Source: three-view drawing plus pictorial views. Frame: mm from the lowest corner of the part. Give positions to 0.01 mm unless a question says otherwise; leave off trailing zeros. Order: outer loops, then holes, each group sorted by start corner. A loop starts at its lowest first (then second) coordinate and runs counter-clockwise, first axis right, second up. Notation, with made-up numbers: M -0.5,69 L 20.5,69 A26 cw 20.5,90 Z; hole C 29.25,7 d3. An arc over 180 degrees is marked long. Use CSV: the item, a comma, the result in double quotes.
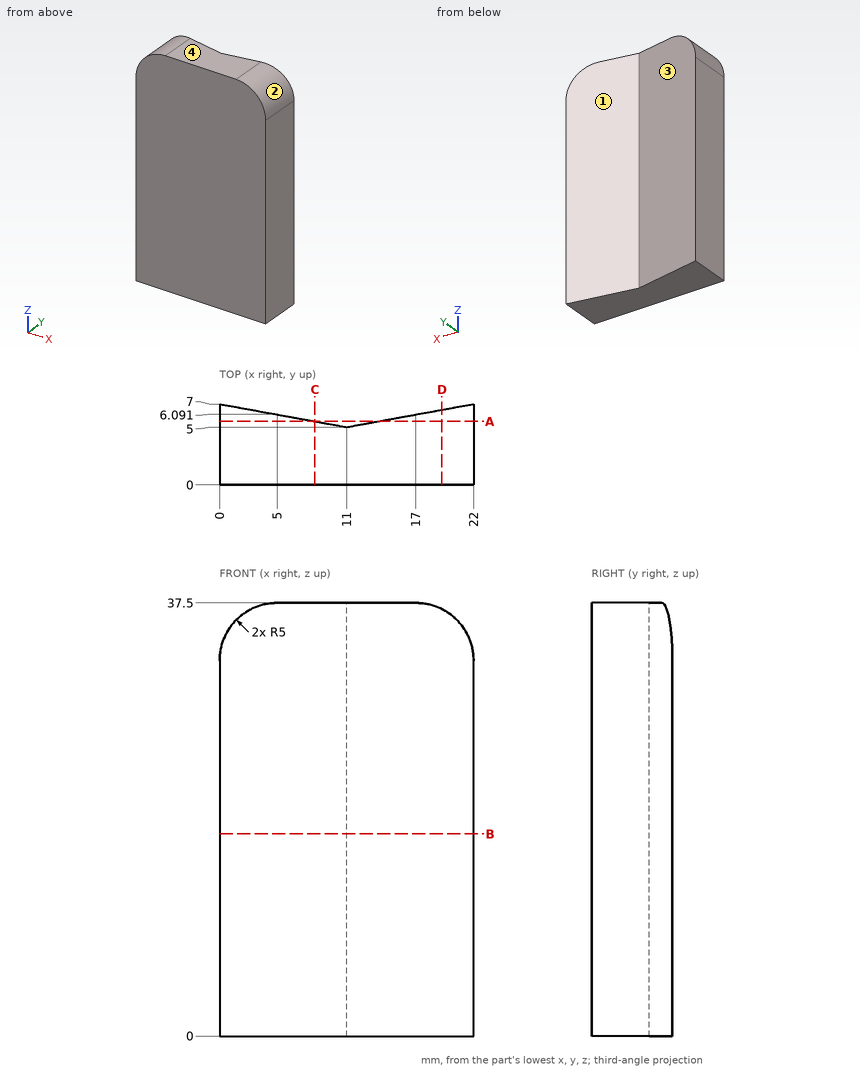
1. Section A-A, the plane y = 5.5. Return the cut outline in (x, z).
Answer:
outline,"M 0,0 L 8.25,0 L 8.25,37.5 L 5,37.5 A5 ccw 0,32.5 Z; M 13.75,0 L 22,0 L 22,32.5 A5 ccw 17,37.5 L 13.75,37.5 Z"
2. Pull-direction query (X, two-part tool) for the marked faces 1, 2, 3 and 4; classes: +X half, -X half, draft (parallel to the pull), parting line (faces both ways), or undercut.
Answer:
face 1,"undercut"
face 2,"+X half"
face 3,"undercut"
face 4,"draft"
3. Section B-B, the plane z = 17.5. Return the cut outline in (x, y).
Answer:
outline,"M 0,0 L 22,0 L 22,7 L 11,5 L 0,7 Z"
4. Line query: line 1 (Y direction, x = 14.5, z = 23.5); line 2 (Y direction, x = 12.75, z = 24); line 3 (Z direction, x = 17.25, y = 0.5). Output: solid intervals per line, ascending.
Answer:
line 1,"0 to 5.64"
line 2,"0 to 5.32"
line 3,"0 to 37.49"
5. Section D-D, the plane x = 19.25. Return the cut outline in (y, z) (3 decimals).
Answer:
outline,"M 0,0 L 6.5,0 L 6.5,36.965 L 0,36.965 Z"
6. Section C-C, the plane x = 8.25. Return the cut outline in (y, z).
Answer:
outline,"M 0,0 L 5.5,0 L 5.5,37.5 L 0,37.5 Z"
